Source: CAD feature listing. Evaluate the final solid. Frame: model axes, mm. Face numbers are marked on the shaded views. Round coordinates to 2 decimals unless told otherwise and drop trailing zeros. Loops run counter-clockwise (first coordinate to the right, second up) from the corner with the lowest first, then second, coordinate; pieces in that order, holes last.
Item 1: Ray query, L1, parallel to Y at x = 0, z = -9.75; L2, parallel to X at y = -2, z = -9.25; L3, parallel to Y at x = 1.75, z = -10.75. Return the intervals inside material, ascending.
Item 2: First-contact query: P1, Ø1, axis at x = -8, z = -7.5, coming from the -Y side; P2, Ø1.5, axis at x = -5, z = -2, coming from the +Y side. Flat tips, straight axial feed; report the tip coordinate or a pass-through.
Item 3: Section query A-A on z = -3. Return loops of the section in (x, y), then the cut area to 3 significant figures.
Item 4: Pull-direction query (Y, two-part tool) for the marked faces 1, 2, 3 and 4; classes: released by +Y, released by -Y, zero draft, split by the parting line, or undercut.
```python
from build123d import *

# Parameters (mm, degrees)
F1_DEPTH = 16
F4_D     = 14


with BuildPart() as f1:
    # F0 (on Top) → F1 (new body)
    with BuildSketch(Plane.XY):
        Polygon((13.509996299, -7.8), (13.509996299, 7.8), (0, 15.6), (-13.509996299, 7.8), (-13.509996299, -7.8), (0, -15.6), align=None)
    extrude(amount=-F1_DEPTH)

    # F2 (on Front) → F3 (revolve, cut)
    with BuildSketch(Plane.XZ):
        Polygon((16, -1.4376021703), (16, 0), (13.51, 0), align=None)
    revolve(axis=Axis((0, 0, -8), (0, 0, -1)), mode=Mode.SUBTRACT)

    # F4 (through all)
    with Locations(Plane.XY):
        with Locations((0, 0)):
            Hole(F4_D / 2)


solid = f1.part
```
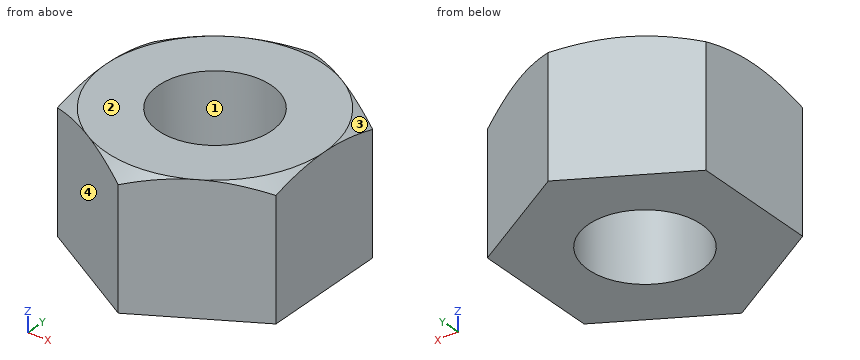
Data:
1. L1: y = -15.6 to -7, 7 to 15.6
1. L2: x = -13.51 to -6.71, 6.71 to 13.51
1. L3: y = -14.59 to -6.78, 6.78 to 14.59
2. P1: stops at y = -11.27
2. P2: stops at y = 13.15
3. outline: (-13.51, -7.8) - (0, -15.6) - (13.51, -7.8) - (13.51, 7.8) - (0, 15.6) - (-13.51, 7.8) - close; hole circle Ø14 at (0, 0)
3. area: 478 mm2
4. face 1: undercut
4. face 2: zero draft
4. face 3: released by +Y
4. face 4: released by -Y
